Geometry check sheet. Reference: the model listing, model coordinates, mm. Face numbers are marked on the shaded views. A direction names the side the tool comes from. Give positions to 0.01 mm unless a question says otherwise; leave off trailing zeros. Write each loop counter-clockwise with the first axis right and the second up, starting at its lowest first coordinate (ties: lowest second). Pieces come first, ordered by that corner, then holes. Notation, with made-up numbers: (-14, -31.75) - (1, -31.75) arc R25 ccw to (1, -1.75) - close; hole circle Ø4 at (6, 28). An arc over 180 degrees is marked (long way). One line per question, with ' | ' between items. Start each with the question number.
Q1. Section check C-C on y = 0.55. Record the boundary of the cut face in (x, z), and give its area (3 significant figures).
Q2. Thickness scan on L1, parallel to X at y = 0.7, z = 0; L2, parallel to Z at x = 0, y = 0.65; L3, parallel to Y at x = -6, z = -9. Record the ranges inside material, lowest first. Write a range as [from, to].
Q3. Set-up check for the marked faces 1 and 2: record each of +Z, -Z, +X, -X, +Y, -Y from which the full face is reachable in a straight line by a thin tool's end or side.
Q4. Gauge pin test, flat ends, axial feed: P1, Ø1.3, axis at x = -14, z = 0, coming from the +Y side; P2, Ø1.9, axis at x = 14, z = 0, coming from the +Y side. Record the tip position at first contact, or that the pin passes through.
Q5. Section check B-B on x = 0. Record the boundary of the cut face in (y, z).
Q6. Section check A-A on z = 0. Record the boundary of the cut face in (x, y).
Q7. Section check D-D on z = 4. Record the boundary of the cut face in (x, y).
```python
from build123d import *

# Parameters (mm, degrees)
SKETCH_1_R          = 16.75
EXTRUDE_1_DEPTH     = 1
SKETCH_2_R          = 10.35
EXTRUDE_2_DEPTH     = 0.65
SKETCH_3_R          = 5.25
CUT_EXTRUDE_1_DEPTH = 2.65
SKETCH_4_R          = 0.7499985
CUT_EXTRUDE_2_DEPTH = 2.65


with BuildPart() as part:
    # Эскиз1 → Бобышка-Вытянуть1 (new body)
    with BuildSketch(Plane(origin=(0, 0, 0), x_dir=(1, 0, 0), z_dir=(0, 1, 0))):
        Circle(SKETCH_1_R)
    extrude(amount=EXTRUDE_1_DEPTH)

    # Эскиз2 → Бобышка-Вытянуть2 (add)
    with BuildSketch(Plane(origin=(0, 1, 0), x_dir=(1, 0, 0), z_dir=(0, 1, 0))):
        Circle(SKETCH_2_R)
    extrude(amount=EXTRUDE_2_DEPTH)

    # Эскиз3 → Вырез-Вытянуть1 (cut, through all)
    with BuildSketch(Plane(origin=(0, 1.65, 0), x_dir=(1, 0, 0), z_dir=(0, 1, 0))):
        Circle(SKETCH_3_R)
    extrude(amount=-CUT_EXTRUDE_1_DEPTH, mode=Mode.SUBTRACT)

    # Эскиз4 → Вырез-Вытянуть2 (cut, through all)
    with BuildSketch(Plane(origin=(0, 0, 0), x_dir=(-1, 0, 0), z_dir=(0, -1, 0))):
        with Locations((-14.0000228, 0)):
            Circle(SKETCH_4_R)
        with Locations((13.999972, 0)):
            Circle(SKETCH_4_R)
    extrude(amount=-CUT_EXTRUDE_2_DEPTH, mode=Mode.SUBTRACT)


solid = part.part
```
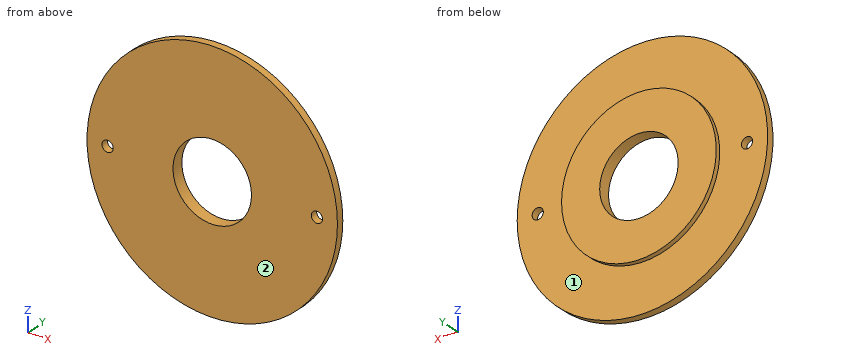
Working result:
1) outline: circle Ø33.5 at (0, 0); hole circle Ø1.5 at (-14, 0); hole circle Ø10.5 at (0, 0); hole circle Ø1.5 at (14, 0) | area: 791 mm2
2) L1: x = [-16.75, -14.75], [-13.25, -5.25], [5.25, 13.25], [14.75, 16.75] | L2: z = [-16.75, -5.25], [5.25, 16.75] | L3: y = [0, 1]
3) face 1: +Y | face 2: +Z, -Z, +X, -X, -Y
4) P1: passes through | P2: stops at y = 1
5) outline: (0, -16.75) - (1, -16.75) - (1, -10.35) - (1.65, -10.35) - (1.65, -5.25) - (0, -5.25) - close; (0, 5.25) - (1.65, 5.25) - (1.65, 10.35) - (1, 10.35) - (1, 16.75) - (0, 16.75) - close
6) outline: (-16.75, 0) - (-14.75, 0) - (-14.75, 1) - (-16.75, 1) - close; (-13.25, 0) - (-5.25, 0) - (-5.25, 1.65) - (-10.35, 1.65) - (-10.35, 1) - (-13.25, 1) - close; (5.25, 0) - (13.25, 0) - (13.25, 1) - (10.35, 1) - (10.35, 1.65) - (5.25, 1.65) - close; (14.75, 0) - (16.75, 0) - (16.75, 1) - (14.75, 1) - close
7) outline: (-16.27, 0) - (-3.4, 0) - (-3.4, 1.65) - (-9.55, 1.65) - (-9.55, 1) - (-16.27, 1) - close; (3.4, 0) - (16.27, 0) - (16.27, 1) - (9.55, 1) - (9.55, 1.65) - (3.4, 1.65) - close
